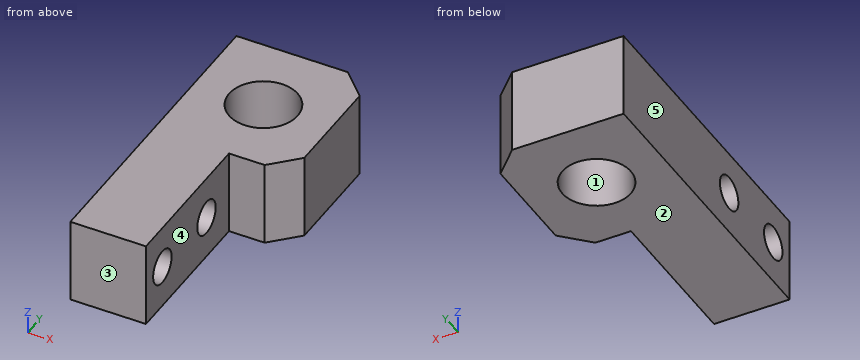
from build123d import *
from OCP.BRepFilletAPI import BRepFilletAPI_MakeChamfer

# Parameters (mm, degrees)
SKETCH_1_W            = 10
SKETCH_1_H            = 36
EXTRUDE_1_DEPTH       = 16
SKETCH_5_R            = 4.000000001
CUT_EXTRUDE_2_DEPTH   = 62.591736841
CUT_EXTRUDE_3_DEPTH   = 62.591736841
CHAMFER_1_SIZE        = 3
CHAMFER_1_SIZE2       = 3.003831905
SKETCH_7_R            = 2
CUT_EXTRUDE_2_2_DEPTH = 63.573848038


with BuildPart() as part:
    # Эскиз1 → Вытянуть1 (new body)
    with BuildSketch(Plane(origin=(0, 0, 0), x_dir=(0, 0, -1), z_dir=(1, 0, 0))):
        with Locations((-15, -40.630555576)):
            Rectangle(SKETCH_1_W, SKETCH_1_H)
    extrude(amount=EXTRUDE_1_DEPTH)

    # Эскиз5 → Cut-Extrude 2 (cut, through all)
    with BuildSketch(Plane.XY.offset(20)):
        with Locations((8, -31.630555576)):
            Circle(SKETCH_5_R)
    extrude(amount=-CUT_EXTRUDE_2_DEPTH, mode=Mode.SUBTRACT)

    # Эскиз6 → Вырез-Вытянуть3 (cut, through all)
    with BuildSketch(Plane.XY.offset(20)):
        Polygon((16, -40.630555576), (16, -58.630555576), (8.828613207, -58.630555576), (8.828613207, -40.639698094), align=None)
    extrude(amount=-CUT_EXTRUDE_3_DEPTH, mode=Mode.SUBTRACT)

    # Фаска1: one chamfer whose edges measure the first distance from different faces: ONE call of the kernel's chamfer builder (chamfer() names one face for all edges)
    chamfer_1_edges_1 = [part.edges().sort_by_distance(p)[0] for p in [
        (16, -40.630555576, 15),
    ]]
    chamfer_1_side_1 = [part.faces().sort_by_distance(p)[0] for p in [
        (16, -31.630555576, 15),
    ]]
    chamfer_1_edges_2 = [part.edges().sort_by_distance(p)[0] for p in [
        (16, -22.630555576, 15),
    ]]
    chamfer_1 = BRepFilletAPI_MakeChamfer(part.part.solid().wrapped)
    for e in chamfer_1_edges_1:
        chamfer_1.Add(CHAMFER_1_SIZE, CHAMFER_1_SIZE2, e.wrapped, chamfer_1_side_1[0].wrapped)  # the first distance lies on this face
    for e in chamfer_1_edges_2:
        chamfer_1.Add(CHAMFER_1_SIZE, e.wrapped)
    add(Compound.cast(chamfer_1.Shape()), mode=Mode.REPLACE)

    # Эскиз7 → Cut-Extrude 2 2 (cut, through all)
    with BuildSketch(Plane(origin=(8.828613207, 0, 0), x_dir=(0, 0, -1), z_dir=(1, 0, 0))):
        with Locations((-15, -55.075818026)):
            Circle(SKETCH_7_R)
        with Locations((-15, -45.513282345)):
            Circle(SKETCH_7_R)
    extrude(amount=-CUT_EXTRUDE_2_2_DEPTH, mode=Mode.SUBTRACT)


solid = part.part
Geometry: final body of the model. Coordinates: model frame, mm. Face numbers are marked on the shaded views. A direction names the side the tool comes from. Round coordinates to 2 decimals unless told otherwise and drop trailing zeros. Loops run counter-clockwise (first coordinate to the right, second up) from the corner with the lowest first, then second, coordinate; pieces in that order, holes last. Notation, with made-up numbers: M 69,85.25 L 127,85.25 A20 ccw 127,95.25 Z; hole C -11,21.25 d5. An arc over 180 degrees is marked long. Put each result on its own line as item: value. Start each with the question number.
(1) Section query D-D (x = 9.75). Return loops of the section in (y, z).
(2) Material intervals for line 1 along Y through (x, z) = (8, 14.75); line 2 along Y through (x, z) = (3.5, 14.75); line 3 along Y through (x, z) = (5.75, 16.75), sorted ascending. Write a range as [from, to].
(3) Draft query along Y for the marked faces 1, 2 and 3. Return one class per face: +Y half, -Y half, draft (parallel to the pull), parting line (faces both ways), or undercut.
(4) Set-up query: the marked faces 4 and 5. Return all of +Z, -Z, +X, -X, +Y, -Y with unobstructed straight access to the full face (end or side cutting, diameter ignored); none if empty.
(5) Section query C-C (z = 15). Return loops of the section in (x, y).
(6) Section query A-A (x = 6). Return loops of the section in (y, z), then the cut area to 3 significant figures.
(7) Section query B-B (y = -34). Return loops of the section in (x, z).
(8) Contact query for a flat-ended pin moving along its axis: pin 1 Ø3 at (y, z) = (-49.5, 17.5) entering from +X. Output: stop coordinate, or through.
Findings below:
1. outline: M -40.64,10 L -35.23,10 L -35.23,20 L -40.64,20 Z; M -28.03,10 L -22.63,10 L -22.63,20 L -28.03,20 Z
2. line 1: y = [-58.63, -57.06], [-53.09, -47.5], [-43.53, -35.63], [-27.63, -22.63]
2. line 2: y = [-58.63, -57.06], [-53.09, -47.5], [-43.53, -22.63]
2. line 3: y = [-58.63, -56.04], [-54.11, -46.48], [-44.55, -34.94], [-28.32, -22.63]
3. face 1: undercut
3. face 2: draft
3. face 3: -Y half
4. face 4: +Z, -Z, +X, -Y
4. face 5: +Z, -Z, -X, +Y, -Y
5. outline: M 0,-58.63 L 8.83,-58.63 L 8.83,-57.08 L 0,-57.08 Z; M 0,-53.08 L 8.83,-53.08 L 8.83,-47.51 L 0,-47.51 Z; M 0,-43.51 L 8.83,-43.51 L 8.83,-40.64 L 13,-40.63 L 16,-37.63 L 16,-25.63 L 13,-22.63 L 0,-22.63 Z; hole C 8,-31.63 d8
6. outline: M -58.63,10 L -35.09,10 L -35.09,20 L -58.63,20 Z; M -28.17,10 L -22.63,10 L -22.63,20 L -28.17,20 Z; hole C -55.08,15 d4; hole C -45.51,15 d4
6. area: 266 mm2
7. outline: M 0,10 L 4.78,10 L 4.78,20 L 0,20 Z; M 11.22,10 L 16,10 L 16,20 L 11.22,20 Z
8. pin 1: stops at x = 8.83
